Source: CAD feature listing. Evaluate the final solid. Frame: model axes, mm. Coordinates: 2 decimals unless noted, no trailing zeros. Order: outer loops, then holes, each group sorted by start corner. A loop starts at its lowest first (then second) coordinate and runs counter-clockwise, first axis right, second up.
```python
from build123d import *

# Parameters (mm, degrees)
SKETCH1_W           = 127
SKETCH1_H           = 19.05
BOSS_EXTRUDE1_DEPTH = 19.05
CUT_EXTRUDE1_REACH  = 111.559
SKETCH2_R           = 2.54
CUT_EXTRUDE2_REACH  = 111.559
SKETCH3_R           = 2.54


with BuildPart() as part:
    # Sketch1 → Boss-Extrude1 (new body)
    with BuildSketch(Plane(origin=(0, 0, 0), x_dir=(1, 0, 0), z_dir=(0, 1, 0))):
        with Locations((-42.694499973, -2.843794964)):
            Rectangle(SKETCH1_W, SKETCH1_H)
    extrude(amount=BOSS_EXTRUDE1_DEPTH)

    # Sketch2 → Cut-Extrude1 (cut, up to next)
    with BuildSketch(Plane.XY.offset(12.368794964), mode=Mode.PRIVATE) as cut_extrude1_sk1:
        with Locations((-4.594499973, 12.7)):
            Circle(SKETCH2_R)
    cut_extrude1_tool1 = extrude(cut_extrude1_sk1.sketch, amount=-CUT_EXTRUDE1_REACH, mode=Mode.PRIVATE) & part.part
    # Sketch2 → Cut-Extrude1 (cut, up to next)
    with BuildSketch(Plane.XY.offset(12.368794964), mode=Mode.PRIVATE) as cut_extrude1_sk2:
        with Locations((-80.794499973, 12.7)):
            Circle(SKETCH2_R)
    cut_extrude1_tool2 = extrude(cut_extrude1_sk2.sketch, amount=-CUT_EXTRUDE1_REACH, mode=Mode.PRIVATE) & part.part
    add(cut_extrude1_tool1.solids().sort_by_distance((-4.5945, 12.7, 12.368795))[0], mode=Mode.SUBTRACT)
    add(cut_extrude1_tool2.solids().sort_by_distance((-80.7945, 12.7, 12.368795))[0], mode=Mode.SUBTRACT)

    # Sketch3 → Cut-Extrude2 (cut, up to next)
    with BuildSketch(Plane(origin=(0, 0, -6.681205036), x_dir=(-1, 0, 0), z_dir=(0, 0, -1)), mode=Mode.PRIVATE) as cut_extrude2_sk1:
        with Locations((95.145499973, 11.176)):
            Circle(SKETCH3_R)
    cut_extrude2_tool1 = extrude(cut_extrude2_sk1.sketch, amount=-CUT_EXTRUDE2_REACH, mode=Mode.PRIVATE) & part.part
    # Sketch3 → Cut-Extrude2 (cut, up to next)
    with BuildSketch(Plane(origin=(0, 0, -6.681205036), x_dir=(-1, 0, 0), z_dir=(0, 0, -1)), mode=Mode.PRIVATE) as cut_extrude2_sk2:
        with Locations((-9.756500027, 11.176)):
            Circle(SKETCH3_R)
    cut_extrude2_tool2 = extrude(cut_extrude2_sk2.sketch, amount=-CUT_EXTRUDE2_REACH, mode=Mode.PRIVATE) & part.part
    add(cut_extrude2_tool1.solids().sort_by_distance((-95.1455, 11.176, -6.681205))[0], mode=Mode.SUBTRACT)
    add(cut_extrude2_tool2.solids().sort_by_distance((9.7565, 11.176, -6.681205))[0], mode=Mode.SUBTRACT)


solid = part.part
```
1. Draft query along Y for faces 1 (the flat face through (20.806, 9, 3)), 2 (the cylindrical face through (-4.925, 15.218, 2.977)), 3 (the flat face through (-44, 0, 3)). Return one class per face: +Y half, -Y half, draft (parallel to the pull), parting line (faces both ways), or undercut.
2. Section query A-A, the plane z = 5.25. Output: boundary loops of the cut face in (x, y).
3. Material intervals for line 1 along X through (y, z) = (14.75, -5.75); line 2 along Y through (x, z) = (9.5, 6.25); line 3 along X through (y, z) = (11.25, 5.5), sorted ascending.
Answer key:
1. face 1: draft
1. face 2: undercut
1. face 3: -Y half
2. outline: (-106.19, 0) - (20.81, 0) - (20.81, 19.05) - (-106.19, 19.05) - close; hole circle Ø5.08 at (-95.15, 11.18); hole circle Ø5.08 at (-80.79, 12.7); hole circle Ø5.08 at (-4.59, 12.7); hole circle Ø5.08 at (9.76, 11.18)
3. line 1: x = -106.19 to -82.29, -79.29 to -6.09, -3.09 to 20.81
3. line 2: y = 0 to 8.65, 13.7 to 19.05
3. line 3: x = -106.19 to -97.68, -92.61 to -82.88, -78.71 to -6.68, -2.51 to 7.22, 12.3 to 20.81
